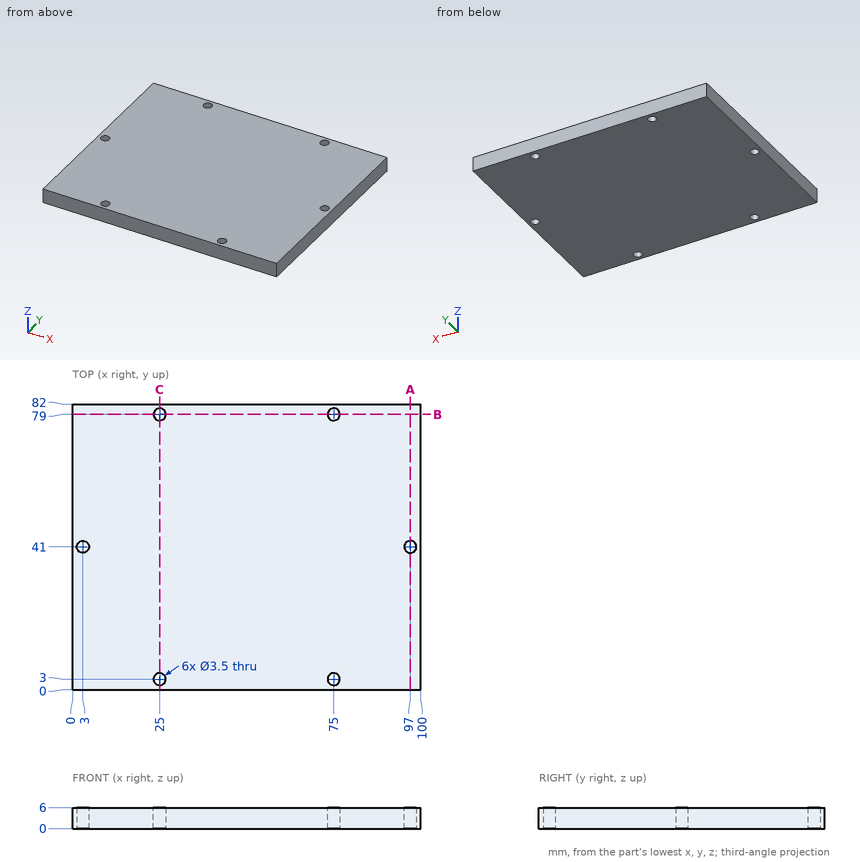
Here's the drawing with two shaded views (mm, measured from the low corner). I have some questions. Give positions to 0.01 mm unless a question says otherwise; leave off trailing zeros. Loops run counter-clockwise (first coordinate to the right, second up) from the corner with the lowest first, then second, coordinate; pieces in that order, holes last. Notation, with made-up numbers: (-32, 25) -> (-22, 25) arc R28 cw to (-22, 44) -> close; hole circle Ø9 at (84, -14). An arc over 180 degrees is marked (long way). One line per item, written item: value.
Q1. Suppose I cut it at C-C on x = 25. Please give me the cut outline in (y, z), then the cut area to 3 significant figures.
Answers follow:
outline: (0, 0) -> (1.25, 0) -> (1.25, 6) -> (0, 6) -> close; (4.75, 0) -> (77.25, 0) -> (77.25, 6) -> (4.75, 6) -> close; (80.75, 0) -> (82, 0) -> (82, 6) -> (80.75, 6) -> close
area: 450 mm^2
Q2. Suppose I cut it at A-A on x = 97. Please give me the cut outline in (y, z), then the cut area to 3 significant figures.
Answers follow:
outline: (0, 0) -> (39.25, 0) -> (39.25, 6) -> (0, 6) -> close; (42.75, 0) -> (82, 0) -> (82, 6) -> (42.75, 6) -> close
area: 471 mm^2
Q3. If I drill on line 1 along Y through (x, z) = (75, 2.95); line 2 along X through (y, z) = (79, 2.3); line 3 along X through (y, z) = (41, 2.6), over which ranges is the centre line in solid material (lowest first)?
Answers follow:
line 1: 0 to 1.25, 4.75 to 77.25, 80.75 to 82
line 2: 0 to 23.25, 26.75 to 73.25, 76.75 to 100
line 3: 0 to 1.25, 4.75 to 95.25, 98.75 to 100
Q4. Suppose I cut it at B-B on y = 79. Please give me the cut outline in (x, z), then the cut area to 3 significant figures.
Answers follow:
outline: (0, 0) -> (23.25, 0) -> (23.25, 6) -> (0, 6) -> close; (26.75, 0) -> (73.25, 0) -> (73.25, 6) -> (26.75, 6) -> close; (76.75, 0) -> (100, 0) -> (100, 6) -> (76.75, 6) -> close
area: 558 mm^2
